Check sheet for the modelled part. Datum: model origin and axes. Units: mm. A direction names the side the tool comes from. Give positions to 0.01 mm unless a question says otherwise; leave off trailing zeros. Write each loop counter-clockwise with the first axis right and the second up, starting at its lowest first coordinate (ties: lowest second). Pieces come first, ordered by that corner, then holes.
Autodesk Inventor part; units mm, degrees
ref_plane "YZ Plane" through (0, 0, 0) normal (1, 0, 0) x (0, 1, 0)
ref_plane "XZ Plane" through (0, 0, 0) normal (0, 1, 0) x (-1, 0, 0)
ref_plane "XY Plane" through (0, 0, 0) normal (0, 0, 1) x (1, 0, 0)
sketch "Esboço1" plane through (0, 0, 0) normal (0, 1, 0) x (-1, 0, 0)
  line L0 (0, 0) -> (0, 2)
  line L1 (0, 2) -> (-10, 2)
  line L2 (-10, 2) -> (-10, 4)
  line L3 (-10, 4) -> (-17.1, 4)
  line L4 (-17.1, 4) -> (-17.1, -6.2)
  line L5 (-17.1, -6.2) -> (-15.5004, -6.2)
  line L6 (-15.5004, -6.2) -> (-14.1, -4.2)
  line L7 (-14.1, -4.2) -> (-15.1, -4.2)
  line L8 (-15.1, -4.2) -> (-15.1, 2)
  line L9 (-15.1, 2) -> (-12, 2)
  line L10 (-12, 2) -> (-12, 0)
  line L11 (-12, 0) -> (0, 0)
  line L12 (-12, 0) -> (-11.1591, 0) construction
  line L13 (-10, 0) -> (-10, -4.2)
  line L14 (-10, -4.2) -> (-12, -4.2)
  line L15 (-12, -4.2) -> (-12, 0)
  line L16 (-11.1591, 0) -> (-10, 0) construction
  dimension "d0" = 2
  dimension "d1" = 55
  dimension "d2" = 10
  dimension "d3" = 6.2
  dimension "d4" = 2
  dimension "d5" = 2
  dimension "d6" = 2
  dimension "d7" = 3.1
  dimension "d8" = 1
  dimension "d10" = 2
  dimension "d11" = 2
  dimension "d12" = 12
  dimension "d25" = 2
extrude "Extrusão1" add sketch "Esboço1" along normal blind 10
sketch "Esboço2" plane through (0, 0, 2) normal (0, 0, 1) x (1, 0, 0)
  line L0 (0, 0) -> (0, 10)
  line L1 (0, 0) -> (10, 0)
  point P0 (5, 5)
  dimension "d15" = 5
  dimension "d16" = 5
hole "Furo1" at (5, 5, 2) direction (0, 0, -1) diameter 2.459 end through all
fillet "Arredondamento1" radius 2 5 edges at (17.1, 5, 4) (10, 5, 4) (0, 10, 1) (0, 0, 1) (10, 5, -4.2)
properties part number "cantoneira"
1) Gauge pin test, flat ends, axial feed: pin 1 (4 mm diameter, centred on x = 10, y = 6, fed in from -Z); pin 2 (0.7 mm diameter, centred on y = 5, z = -1, fed in from -X); pin 3 (2 mm diameter, centred on x = 5, y = 5, fed in from -Z); pin 4 (3 mm diameter, centred on x = 2.5, y = 1.5, fed in from -Z). Record the tip position at first contact, or that the pin passes through.
2) Sectioned sample at D-D on z = 1.75. Record the boundary of the cut face in (x, y).
3) Sectioned sample at A-A on x = 5. Record the boundary of the cut face in (y, z), then the cut area to 3 significant figures.
4) Draft check along X on faces 1 (the flat face through (6, 6, 0)), 2 (the flat face through (14.6, 4.9, -4.2)), 3 (the cylindrical face through (16.5, 5.07, 3.43)). Enter one of: +X half, -X half, draft (parallel to the pull), parting line (faces both ways), or undercut.
5) Sectioned sample at B-B on z = -2. Record the boundary of the cut face in (x, y).
6) Access from +Z, -Z, +X, -X, +Y, -Y to the whole of each face (thin tool, end or side, straight path). Record for faces 4 (the flat face through (10, 5, -1)), 5 (the flat face through (14, 5, 2)), 6 (the flat face through (12, 5, -1)).
7) Scan lines: L1, parallel to X at y = 5, z = 0.4; L2, parallel to Y at x = 5, z = 1.25; L3, parallel to Z at x = 1.5, y = 4. Record each from-to range of solid material in increasing order.
Answers below:
1. pin 1: stops at z = -4.2
1. pin 2: stops at x = 10
1. pin 3: passes through
1. pin 4: stops at z = 0
2. outline: (0, 2) arc R2 ccw to (2, 0) - (12, 0) - (12, 10) - (2, 10) arc R2 ccw to (0, 8) - close; (15.1, 0) - (17.1, 0) - (17.1, 10) - (15.1, 10) - close; hole circle Ø2.46 at (5, 5)
3. outline: (0, 0) - (3.77, 0) - (3.77, 2) - (0, 2) - close; (6.23, 0) - (10, 0) - (10, 2) - (6.23, 2) - close
3. area: 15.1 mm2
4. face 1: draft
4. face 2: undercut
4. face 3: +X half
5. outline: (10, 0) - (12, 0) - (12, 10) - (10, 10) - close; (15.1, 0) - (17.1, 0) - (17.1, 10) - (15.1, 10) - close
6. face 4: -Z, -X, +Y, -Y
6. face 5: +Y, -Y
6. face 6: -Z, +Y, -Y
7. L1: x = 0 to 3.77, 6.23 to 12, 15.1 to 17.1
7. L2: y = 0 to 3.77, 6.23 to 10
7. L3: z = 0 to 2
